Can you work these out from the model? Positions are in its coordinate system, mm. A direction names the side the tool comes from. Coordinates: 2 decimals unless noted, no trailing zeros. Write each loop counter-clockwise with the first axis right and the second up, starting at its lowest first coordinate (ties: lowest second). Pieces come first, ordered by that corner, then holes. Notation, with made-up numbers: (59.5, 23.25) - (76.5, 23.25) arc R21 cw to (76.5, 48.25) - close; hole circle Ø9 at (-15, 62). An arc over 180 degrees is marked (long way). Use one line per item in the form item = value. Start each with the question number.
(1) If I drill on probe 1 along X at (y, z) = (0, 0.9); probe 2 along Y at (x, z) = (19, 5); probe 3 along Y at (x, z) = (-19, 14.25), over which ranges is the centre line in solid material (lowest first)? Write a range as from..to.
(2) On a 3-axis mill with a long thin cutter (end or side, diameter ignored), from which of +Z, -Z, +X, -X, +Y, -Y can I reach the whole of each face in a straight line? I mean faces 4 (the face through (28.45, 12.05, 1.52)), 5 (the face through (39, 0, 5)), 6 (the face through (26, 8, 3)), 7 (the face through (20.22, -16.32, 4.25)), 8 (the face through (-20.4, 17.56, 13.38)). Say none if no direction works.
(3) Thinking about a two-plate mould opening in Z: for faces 1 (the face through (-19, 18, 5)), 2 (the face through (24.75, 5, 5)), 3 (the face through (-1, 0, 0)), which applies, pulls with the +Z half, pulls with the -Z half, needs draft (parallel to the pull), parting line crosses it, or undercut?
(4) If we section it at B-B on x = -19: Please give me the cut outline in (y, z), then the cut area to 3 significant figures.
(5) If we section it at C-C on z = 12.5: Please give me the cut outline in (x, y), then the cut area to 3 significant figures.
(6) For pin 1 Ø4 at (x, y) = (-9, 14.5) entering from +Z; pin 2 Ø6 at (x, y) = (-29, 6) entering from +Z; pin 3 Ø6 at (x, y) = (-28.5, 0) entering from -Z, each with a flat end and sliding along its axis, tell me the tip position at first contact or that it passes through.
(7) If we section it at D-D on y = 17.5: Please give me the cut outline in (x, z), then the cut area to 3 significant figures.
(8) If we section it at A-A on x = 28.5: Please give me the cut outline in (y, z), then the cut area to 3 significant figures.
```python
from build123d import *
from OCP.BRepFilletAPI import BRepFilletAPI_MakeChamfer

# Parameters (mm, degrees)
SKETCH1_W           = 78
SKETCH1_H           = 50
BOSS_EXTRUDE1_DEPTH = 10
SKETCH3_R           = 4.4
SKETCH3_R_2         = 1.4
BOSS_EXTRUDE2_DEPTH = 15
CUT_EXTRUDE2_START  = -5
SKETCH4_R           = 1.4
CUT_EXTRUDE2_DEPTH  = 5
SKETCH5_R           = 1.4
CUT_EXTRUDE3_DEPTH  = 35
CHAMFER1_SIZE       = 3
CHAMFER1_SIZE2      = 0.528980942
CHAMFER2_SIZE       = 6.994614872
CHAMFER2_SIZE_2     = 15
CUT_EXTRUDE4_START  = -3
CUT_EXTRUDE4_DEPTH  = 3.5
CUT_EXTRUDE5_START  = -3
CUT_EXTRUDE5_DEPTH  = 3


# Read off the part's stored shape, not the designer's step: Cut-Extrude5
with BuildPart() as part:
    # Sketch1 → Boss-Extrude1 (new body)
    with BuildSketch(Plane.XY):
        Rectangle(SKETCH1_W, SKETCH1_H)
    extrude(amount=BOSS_EXTRUDE1_DEPTH)

    # Sketch3 → Boss-Extrude2 (add)
    # profile 1 of 2: a face of its own
    with BuildSketch(Plane.XY.offset(10)):
        with Locations(Location((-19, 17.5, 0), (0, 0, 180))):
            Circle(SKETCH3_R)
        with Locations((-19, 17.5)):
            Circle(SKETCH3_R_2, mode=Mode.SUBTRACT)
    # profile 2 of 2: a face of its own
    with BuildSketch(Plane.XY.offset(10)):
        with Locations(Location((-19, -17.5, 0), (0, 0, 180))):
            Circle(SKETCH3_R)
        with Locations((-19, -17.5)):
            Circle(SKETCH3_R_2, mode=Mode.SUBTRACT)
    extrude(amount=BOSS_EXTRUDE2_DEPTH)

    # Sketch4 → Cut-Extrude2 (cut)
    with BuildSketch(Plane.XY.offset(10).offset(CUT_EXTRUDE2_START)):
        with Locations((-19, 17.5)):
            Circle(SKETCH4_R)
        with Locations((-19, -17.5)):
            Circle(SKETCH4_R)
    extrude(amount=CUT_EXTRUDE2_DEPTH, mode=Mode.SUBTRACT)

    # Sketch5 → Cut-Extrude3 (cut)
    with BuildSketch(Plane(origin=(39, 0, 0), x_dir=(0, 0, -1), z_dir=(1, 0, 0))):
        with Locations((-5, 17.5)):
            Circle(SKETCH5_R)
        with Locations((-5, -17.5)):
            Circle(SKETCH5_R)
    extrude(amount=-CUT_EXTRUDE3_DEPTH, mode=Mode.SUBTRACT)

    # Chamfer1: one chamfer whose edges measure the first distance from different faces: ONE call of the kernel's chamfer builder (chamfer() names one face for all edges)
    chamfer1_edges_1 = [part.edges().sort_by_distance(p)[0] for p in [
        (-20.4, -17.5, 25),
    ]]
    chamfer1_side_1 = [part.faces().sort_by_distance(p)[0] for p in [
        (-20.4, -17.5, 15),
    ]]
    chamfer1_edges_2 = [part.edges().sort_by_distance(p)[0] for p in [
        (-20.4, 17.5, 25),
    ]]
    chamfer1_side_2 = [part.faces().sort_by_distance(p)[0] for p in [
        (-20.4, 17.5, 15),
    ]]
    chamfer1_edges_3 = [part.edges().sort_by_distance(p)[0] for p in [
        (39, 17.5, 6.4),
    ]]
    chamfer1_side_3 = [part.faces().sort_by_distance(p)[0] for p in [
        (21.5, 17.5, 6.4),
    ]]
    chamfer1_edges_4 = [part.edges().sort_by_distance(p)[0] for p in [
        (39, -17.5, 6.4),
    ]]
    chamfer1_side_4 = [part.faces().sort_by_distance(p)[0] for p in [
        (21.5, -17.5, 6.4),
    ]]
    chamfer1 = BRepFilletAPI_MakeChamfer(part.part.solid().wrapped)
    for e in chamfer1_edges_1:
        chamfer1.Add(CHAMFER1_SIZE, CHAMFER1_SIZE2, e.wrapped, chamfer1_side_1[0].wrapped)  # the first distance lies on this face
    for e in chamfer1_edges_2:
        chamfer1.Add(CHAMFER1_SIZE, CHAMFER1_SIZE2, e.wrapped, chamfer1_side_2[0].wrapped)  # the first distance lies on this face
    for e in chamfer1_edges_3:
        chamfer1.Add(CHAMFER1_SIZE, CHAMFER1_SIZE2, e.wrapped, chamfer1_side_3[0].wrapped)  # the first distance lies on this face
    for e in chamfer1_edges_4:
        chamfer1.Add(CHAMFER1_SIZE, CHAMFER1_SIZE2, e.wrapped, chamfer1_side_4[0].wrapped)  # the first distance lies on this face
    add(Compound.cast(chamfer1.Shape()), mode=Mode.REPLACE)

    # Chamfer2
    # the kernel refuses this chamfer: 15, 6.994614872 mm, written as the material it adds along each edge
    with BuildSketch(Plane(origin=(-19, 17.5, 10), x_dir=(-1, 0, 0), z_dir=(0, 1, 0))) as chamfer2_piece_1_section:
        Polygon((4.4 + CHAMFER2_SIZE, 0), (4.4, CHAMFER2_SIZE_2), (4.4, 0), align=None)
    chamfer2_piece_1 = revolve(axis=Axis((-19, 17.5, 10), (0, 0, 1)), mode=Mode.PRIVATE)
    chamfer2_piece_1 = split(chamfer2_piece_1, bisect_by=Plane(origin=(-11.096055179, 25, 17.172081688), z_dir=(0, -1, 0)), keep=Keep.TOP, mode=Mode.PRIVATE)
    chamfer2_piece_1 = split(chamfer2_piece_1, bisect_by=Plane(origin=(-11.096055179, 17.5, 25), z_dir=(0, 0, -1)), keep=Keep.TOP, mode=Mode.PRIVATE)
    add(chamfer2_piece_1)
    with BuildSketch(Plane(origin=(-19, -17.5, 10), x_dir=(-1, 0, 0), z_dir=(0, 1, 0))) as chamfer2_piece_2_section:
        Polygon((4.4 + CHAMFER2_SIZE, 0), (4.4, CHAMFER2_SIZE_2), (4.4, 0), align=None)
    chamfer2_piece_2 = revolve(axis=Axis((-19, -17.5, 10), (0, 0, 1)), mode=Mode.PRIVATE)
    chamfer2_piece_2 = split(chamfer2_piece_2, bisect_by=Plane(origin=(-11.096055179, -25, 17.172081688), z_dir=(0, 1, 0)), keep=Keep.TOP, mode=Mode.PRIVATE)
    chamfer2_piece_2 = split(chamfer2_piece_2, bisect_by=Plane(origin=(-11.096055179, -17.5, 25), z_dir=(0, 0, -1)), keep=Keep.TOP, mode=Mode.PRIVATE)
    add(chamfer2_piece_2)

    # Sketch6 → Cut-Extrude4 (cut)
    with BuildSketch(Plane(origin=(0, 0, 0), x_dir=(-1, 0, 0), z_dir=(0, 0, -1)).offset(CUT_EXTRUDE4_START)):
        with BuildLine():
            Line((-24.75, 10), (-24.75, 0))
            ThreePointArc((-24.75, 0), (-28.5, -3.75), (-32.25, 0))
            Line((-32.25, 0), (-32.25, 10))
            ThreePointArc((-32.25, 10), (-28.5, 13.75), (-24.75, 10))
        make_face()
        with BuildLine():
            Line((24.75, 10), (24.75, 0))
            ThreePointArc((24.75, 0), (28.5, -3.75), (32.25, 0))
            Line((32.25, 0), (32.25, 10))
            ThreePointArc((32.25, 10), (28.5, 13.75), (24.75, 10))
        make_face()
    extrude(amount=-CUT_EXTRUDE4_DEPTH, mode=Mode.SUBTRACT)

    # Cut-Extrude5 outline → Cut-Extrude5 (cut)
    with BuildSketch(Plane(origin=(0, 0, 0), x_dir=(-1, 0, 0), z_dir=(0, 0, -1)).offset(CUT_EXTRUDE5_START)):
        with BuildLine():
            ThreePointArc((26.45, 4.478839135), (26.254757862, 3.41425784), (25.694444444, 2.488243964))
            ThreePointArc((25.694444444, 2.488243964), (28.5, -3.75), (31.305555556, 2.488243964))
            ThreePointArc((31.305555556, 2.488243964), (30.745242138, 3.41425784), (30.55, 4.478839135))
            Line((30.55, 4.478839135), (30.55, 10))
            ThreePointArc((30.55, 10), (28.5, 12.05), (26.45, 10))
            Line((26.45, 10), (26.45, 4.478839135))
        make_face()
        with BuildLine():
            ThreePointArc((-25.694444444, 2.488243964), (-26.254757862, 3.41425784), (-26.45, 4.478839135))
            Line((-26.45, 4.478839135), (-26.45, 10))
            ThreePointArc((-26.45, 10), (-28.5, 12.05), (-30.55, 10))
            Line((-30.55, 10), (-30.55, 4.478839135))
            ThreePointArc((-30.55, 4.478839135), (-30.745242138, 3.41425784), (-31.305555556, 2.488243964))
            ThreePointArc((-31.305555556, 2.488243964), (-28.5, -3.75), (-25.694444444, 2.488243964))
        make_face()
    extrude(amount=CUT_EXTRUDE5_DEPTH, mode=Mode.SUBTRACT)


solid = part.part
```
Reported:
q1.probe_1 = -39..-32.25, -24.75..24.75, 32.25..39
q1.probe_2 = -25..-18.9, -16.1..16.1, 18.9..25
q1.probe_3 = -25..-18.9, -16.1..-8.09, 8.09..16.1, 18.9..25
q2.face_4 = -Z
q2.face_5 = +Z, -Z, +X, +Y, -Y
q2.face_6 = none
q2.face_7 = +X
q2.face_8 = +Z
q3.face_1 = pulls with the +Z half
q3.face_2 = undercut
q3.face_3 = pulls with the -Z half
q4.outline = (-25, 0) - (25, 0) - (25, 18.35) - (21.9, 25) - (19.43, 25) - (18.9, 22) - (18.9, 5) - (16.1, 5) - (16.1, 22) - (15.57, 25) - (13.1, 25) - (6.11, 10) - (-6.11, 10) - (-13.1, 25) - (-15.57, 25) - (-16.1, 22) - (-16.1, 5) - (-18.9, 5) - (-18.9, 22) - (-19.43, 25) - (-21.9, 25) - (-25, 18.35) - close
q4.area = 826 mm2
q5.outline = (-25.96, -25) - (-12.04, -25) arc R10.23 ccw (long way) to start; (-25.96, 25) arc R10.23 ccw (long way) to (-12.04, 25) - close; hole circle Ø2.8 at (-19, -17.5); hole circle Ø2.8 at (-19, 17.5)
q5.area = 593 mm2
q6.pin_1 = 16.34
q6.pin_2 = 10
q6.pin_3 = 6.5
q7.outline = (-39, 0) - (39, 0) - (39, 3.07) - (36, 3.6) - (4, 3.6) - (4, 6.4) - (36, 6.4) - (39, 6.93) - (39, 10) - (-7.61, 10) - (-14.6, 25) - (-17.07, 25) - (-17.6, 22) - (-17.6, 5) - (-20.4, 5) - (-20.4, 22) - (-20.93, 25) - (-23.4, 25) - (-30.39, 10) - (-39, 10) - close
q7.area = 860 mm2
q8.outline = (-25, 0) - (-3.75, 0) - (-3.75, 6.5) - (13.75, 6.5) - (13.75, 3) - (12.05, 3) - (12.05, 0) - (25, 0) - (25, 10) - (-25, 10) - close; hole circle Ø2.8 at (-17.5, 5); hole circle Ø2.8 at (17.5, 5)
q8.area = 379 mm2
